```python
from build123d import *

# Parameters (mm, degrees)
F0_R      = 19.05
F1_DEPTH  = 54.864
F3_W      = 76.2
F3_H      = 29.464
F4_DEPTH  = 82.551
F9_R      = 1.9939
F10_DEPTH = 25.401
F11_R     = 1.9939
F12_DEPTH = 67.921568
F13_R     = 1.9939
F14_DEPTH = 67.921568
F17_DEPTH = 42.164


with BuildPart() as f1:
    # F0 (on Front) → F1 (new body)
    with BuildSketch(Plane.XZ):
        with BuildLine():
            Line((38.1, 0), (15.24, 49.53))
            ThreePointArc((15.24, 49.53), (0, 95.25), (-15.24, 49.53))
            Line((-15.24, 49.53), (-38.1, 0))
            Line((-38.1, 0), (38.1, 0))
        make_face()
        with Locations((0, 69.85)):
            Circle(F0_R, mode=Mode.SUBTRACT)
    extrude(amount=-F1_DEPTH)

    # F3 (on offset) → F4 (cut, through all)
    with BuildSketch(Plane.XY.offset(12.7)):
        with Locations((0, 27.432)):
            Rectangle(F3_W, F3_H)
    extrude(amount=F4_DEPTH, mode=Mode.SUBTRACT)

    # F9 (on face) → F10 (cut, through all)
    with BuildSketch(Plane.XY.offset(69.85)):
        with Locations((0, 6.35)):
            Circle(F9_R)
        with Locations((0, 48.514)):
            Circle(F9_R)
    extrude(amount=F10_DEPTH, mode=Mode.SUBTRACT)

    # F11 (on face) → F12 (cut, through all)
    with BuildSketch(Plane(origin=(30.245937, 0, 17.4625), x_dir=(0, 1, 0), z_dir=(0.866025, 0, 0.5))):
        with Locations((6.35, 60.491874)):
            Circle(F11_R)
        with Locations((48.514, 60.491874)):
            Circle(F11_R)
    extrude(amount=-F12_DEPTH, mode=Mode.SUBTRACT)

    # F13 (on face) → F14 (cut, through all)
    with BuildSketch(Plane(origin=(-30.245937, 0, 17.4625), x_dir=(0, -1, 0), z_dir=(-0.866025, 0, 0.5))):
        with Locations((-48.514, 60.491874)):
            Circle(F13_R)
        with Locations((-6.35, 60.491874)):
            Circle(F13_R)
    extrude(amount=-F14_DEPTH, mode=Mode.SUBTRACT)

    # F16 (on face) → F17 (join, through all)
    with BuildSketch(Plane.XZ):
        with BuildLine():
            Line((-12.497391, 55.472319), (-15.24, 49.53))
            Line((-15.24, 49.53), (-38.1, 0))
            Line((-38.1, 0), (38.1, 0))
            Line((38.1, 0), (15.24, 49.53))
            Line((15.24, 49.53), (12.497391, 55.472319))
            ThreePointArc((12.497391, 55.472319), (0, 50.8), (-12.497391, 55.472319))
        make_face()
    extrude(amount=-F17_DEPTH)


solid = f1.part
```
Verification items for the finished model (mm, model axes). A direction names the side the tool comes from. Coordinates: 2 decimals unless noted, no trailing zeros. Order: outer loops, then holes, each group sorted by start corner. A loop starts at its lowest first (then second) coordinate and runs counter-clockwise, first axis right, second up. Notation, with made-up numbers: (-34, 55.25) - (22, 55.25) arc R16 ccw to (22, 82.25) - close; hole circle Ø11 at (57, 85). An arc over 180 degrees is marked (long way). Return JSON: item names as keys, results as strings.
(1) Thickness scan on line 1 along Y through (x, z) = (0, 91.25); line 2 along Z through (x, y) = (0, 51.5); line 3 along X through (y, z) = (46, 69). Record the ranges inside material, lowest first.
Filled sheet:
{"line 1": "y = 0 to 4.36, 8.34 to 12.7, 42.16 to 46.52, 50.51 to 54.86", "line 2": "z = 0 to 50.8, 88.9 to 95.25", "line 3": "x = -25.39 to -19.03, 19.03 to 25.39"}
(2) Mould release check, pull along Y, two halves, no side actions. Record for faces 1 (the flat face through (-1, 54.864, 38)), 2 (the flat face through (-1, 27, 0)), 3 (the cylindrical face through (1.072, 8.031, 91.977)): pulls with the +Y half, pulls with the -Y half, needs draft (parallel to the pull), parting line crosses it, or undercut.
Filled sheet:
{"face 1": "pulls with the +Y half", "face 2": "needs draft", "face 3": "undercut"}
(3) Go/stop test with flat-tipped pins: pin 1 (1 mm diameter, centred on y = 8.5, z = 49.5, fed in from +X); pin 2 (1 mm diameter, centred on x = 19, y = 13.5, fed in from +Z); pin 3 (12 mm diameter, centred on y = 8.5, z = 68.5, fed in from -X); pin 4 (10 mm diameter, centred on x = -15, z = 68, fed in from -Y). Record where each tip stops, or that it passes through.
Filled sheet:
{"pin 1": "stops at x = 15.85", "pin 2": "stops at z = 42.47", "pin 3": "stops at x = -25.4", "pin 4": "stops at y = 0"}
(4) Section check D-D, the plane y = 18. Record the cut outline in (x, z).
Filled sheet:
{"outline": "(-38.1, 0) - (38.1, 0) - (12.5, 55.47) arc R19.05 cw to (-12.5, 55.47) - close"}
(5) Section check B-B, the plane z = 69.85. Record the cut outline in (x, y).
Filled sheet:
{"outline": "(-25.4, 0) - (-19.05, 0) - (-19.05, 12.7) - (-25.4, 12.7) - close; (-25.4, 42.16) - (-19.05, 42.16) - (-19.05, 54.86) - (-25.4, 54.86) - close; (19.05, 0) - (25.4, 0) - (25.4, 12.7) - (19.05, 12.7) - close; (19.05, 42.16) - (25.4, 42.16) - (25.4, 54.86) - (19.05, 54.86) - close"}
(6) Section check A-A, the plane x = 0. Record the cut outline in (y, z).
Filled sheet:
{"outline": "(0, 0) - (54.86, 0) - (54.86, 50.8) - (0, 50.8) - close; (0, 88.9) - (4.36, 88.9) - (4.36, 95.25) - (0, 95.25) - close; (8.34, 88.9) - (12.7, 88.9) - (12.7, 95.25) - (8.34, 95.25) - close; (42.16, 88.9) - (46.52, 88.9) - (46.52, 95.25) - (42.16, 95.25) - close; (50.51, 88.9) - (54.86, 88.9) - (54.86, 95.25) - (50.51, 95.25) - close"}
(7) Access from +Z, -Z, +X, -X, +Y, -Y to the whole of each face (thin tool, end or side, straight path). Record for faces 4 (the cylindrical face through (18.78, 4.51, 58.12)), 5 (the cylindrical face through (-0.432, 46.568, 91.977)).
Filled sheet:
{"face 4": "none", "face 5": "+Z"}
(8) Section check C-C, the plane y = 10.5. Record the cut outline in (x, z).
Filled sheet:
{"outline": "(-38.1, 0) - (38.1, 0) - (15.24, 49.53) arc R25.4 ccw (long way) to (-15.24, 49.53) - close; hole circle Ø38.1 at (0, 69.85)"}
